Verification items for the finished model (mm, model axes). A direction names the side the tool comes from. Round coordinates to 2 decimals unless told otherwise and drop trailing zeros. Loops run counter-clockwise (first coordinate to the right, second up) from the corner with the lowest first, then second, coordinate; pieces in that order, holes last. Notation, with made-up numbers: (67, -25) -> (116, -25) arc R17 ccw to (116, -6) -> close; hole circle Ø8 at (5.5, 76.5). An arc over 180 degrees is marked (long way). Write item = value, one per line. Start each with the question number.
Autodesk Inventor part; units mm, degrees
ref_plane "Work Plane1" through (-19.935, -55, 0) normal (0, -1, 0) x (1, 0, 0)
ref_plane "YZ Plane" through (0, 0, 0) normal (1, 0, 0) x (0, 1, 0)
ref_plane "XZ Plane" through (0, 0, 0) normal (0, 1, 0) x (-1, 0, 0)
sketch "Sketch1" plane through (0, 0, 0) normal (0, 0, 1) x (1, 0, 0)
  line L0 (-51, 56) -> (51, 56)
  line L1 (51, 56) -> (51, -56)
  line L2 (51, -56) -> (-51, -56)
  line L3 (-51, -56) -> (-51, 56)
  line L4 (-51, 56) -> (51, -56) construction
  line L5 (51, 56) -> (-51, -56) construction
  point P0 (0, 0)
  point P1 (0, 0)
  point P2 (0, 0)
  dimension "d0" = 102
  dimension "d1" = 112
extrude "Extrusion1" add sketch "Sketch1" along normal blind 3
sketch "Sketch2" plane through (0, 0, 3) normal (0, 0, 1) x (1, 0, 0)
  line L0 (-51, -56) -> (51, -56)
  line L1 (-30.065, -59) -> (-19.935, -59)
  line L2 (-19.935, -59) -> (-19.935, -56)
  line L3 (-19.935, -56) -> (-30.065, -56)
  line L4 (-30.065, -56) -> (-30.065, -59)
  line L5 (-30.065, -59) -> (-19.935, -56) construction
  line L6 (-19.935, -59) -> (-30.065, -56) construction
  line L7 (19.935, -59) -> (30.065, -59)
  line L8 (30.065, -59) -> (30.065, -56)
  line L9 (30.065, -56) -> (19.935, -56)
  line L10 (19.935, -56) -> (19.935, -59)
  line L11 (19.935, -59) -> (30.065, -56) construction
  line L12 (30.065, -59) -> (19.935, -56) construction
  point P0 (0, 0)
  point P1 (-25, -57.5)
  point P2 (25, -57.5)
  dimension "d4" = 3
  dimension "d5" = 25
  dimension "d6" = 25
  dimension "d7" = 10.13
  dimension "d8" = 10.13
extrude "Extrusion2" add sketch "Sketch2" against normal blind 3
mirror "Mirror1" about plane through (0, 0, 0) normal (0, 1, 0) of "Extrusion2"
sketch "Sketch3" plane through (0, 0, 0) normal (0, 0, -1) x (-1, 0, 0)
  line L0 (-51, -56) -> (-51, 56) construction
  line L1 (-51, 55) -> (51, 55) construction
  line L2 (51, 56) -> (51, -56) construction
  line L3 (-51, -55) -> (51, -55) construction
  line L4 (-19.935, -56) -> (19.935, -56) construction
  line L5 (-30.065, 56) -> (-51, 56) construction
  point P0 (0, 0)
  dimension "d11" = 1
  dimension "d12" = 1
ref_plane "Work Plane1" through (-19.935, -55, 0) normal (0, -1, 0) x (1, 0, 0)
sketch "Sketch4" plane through (0, 0, 3) normal (0, 0, 1) x (1, 0, 0)
  line L0 (-51, 56) -> (-51, -56)
  line L1 (-51, -56) -> (-30.065, -56)
  line L2 (-30.065, 56) -> (-51, 56)
  line L3 (51, -56) -> (51, 56)
  point P0 (0, 0)
  point P1 (-40.9, -50.9)
  point P2 (-40.9, 50.9)
  point P3 (41.9, -50.9)
  point P4 (40.9, 50.9)
  dimension "d14" = 10.1
  dimension "d15" = 5.1
  dimension "d16" = 5.1
  dimension "d17" = 9.1
  dimension "d32" = 10.1
hole "Hole2" at (-40.9, -50.9, 3) at (41.9, -50.9, 3) at (40.9, 50.9, 3) at (-40.9, 50.9, 3) direction (0, 0, -1) diameter 3 end through all
equation "\"d8\" = d7"
equation "\"d12\" = d11"
equation "\"kerf\" = 0.13"
properties part number "BottomPlate" material "Acrylic, Clear"
(1) Depth check by flat-ended pin: pin 1 Ø1.5 at (y, z) = (58, 2) entering from -X (3 decimals); pin 2 Ø1.5 at (x, z) = (2.5, 1) entering from +Y; pin 3 Ø0.9 at (y, z) = (58, 1) entering from +X (3 decimals). Enter the tip coordinate at first touch or a pass-through.
(2) Scan lines: line 1 (Y direction, x = -40.9, z = 1.55); line 2 (X direction, y = -50.9, z = 1.75); line 3 (X direction, y = 50.9, z = 1.7). Record each from-to range of solid material in increasing order. Write a range as [from, to].
(3) Section check A-A on y = 50.9. Enter the section's corners in (x, z).
(4) Draft check along X on faces 4 (the flat face through (25, -59, 2)), 5 (the flat face through (19.935, 58, 2)), 6 (the flat face through (30.065, -58, 2)). Enter one of: +X half, -X half, draft (parallel to the pull), parting line (faces both ways), or undercut.
(5) Access from +Z, -Z, +X, -X, +Y, -Y to the whole of each face (thin tool, end or side, straight path). Record for faces 1 (the flat face through (30.065, 57, 2)), 2 (the flat face through (-40, -56, 1)), 3 (the flat face through (0, 56, 1)).
(6) Section check B-B on x = -40.9. Enter the section's corners in (y, z).
(7) Section check C-C on z = 0.7. Enter the section's corners in (x, y) (3 decimals).
Computed values:
q1.pin_1 = -30.065
q1.pin_2 = 56
q1.pin_3 = 30.065
q2.line_1 = [-56, -52.4], [-49.4, 49.4], [52.4, 56]
q2.line_2 = [-51, -42.4], [-39.4, 40.4], [43.4, 51]
q2.line_3 = [-51, -42.4], [-39.4, 39.4], [42.4, 51]
q3.outline = (-51, 0) -> (-42.4, 0) -> (-42.4, 3) -> (-51, 3) -> close; (-39.4, 0) -> (39.4, 0) -> (39.4, 3) -> (-39.4, 3) -> close; (42.4, 0) -> (51, 0) -> (51, 3) -> (42.4, 3) -> close
q4.face_4 = draft
q4.face_5 = undercut
q4.face_6 = +X half
q5.face_1 = +Z, -Z, +X, +Y
q5.face_2 = +Z, -Z, -X, -Y
q5.face_3 = +Z, -Z, +Y
q6.outline = (-56, 0) -> (-52.4, 0) -> (-52.4, 3) -> (-56, 3) -> close; (-49.4, 0) -> (49.4, 0) -> (49.4, 3) -> (-49.4, 3) -> close; (52.4, 0) -> (56, 0) -> (56, 3) -> (52.4, 3) -> close
q7.outline = (-51, -56) -> (-30.065, -56) -> (-30.065, -59) -> (-19.935, -59) -> (-19.935, -56) -> (19.935, -56) -> (19.935, -59) -> (30.065, -59) -> (30.065, -56) -> (51, -56) -> (51, 56) -> (30.065, 56) -> (30.065, 59) -> (19.935, 59) -> (19.935, 56) -> (-19.935, 56) -> (-19.935, 59) -> (-30.065, 59) -> (-30.065, 56) -> (-51, 56) -> close; hole circle Ø3 at (-40.9, -50.9); hole circle Ø3 at (-40.9, 50.9); hole circle Ø3 at (40.9, 50.9); hole circle Ø3 at (41.9, -50.9)
